Build history of the part. All positions in model axes, mm. Face numbers are marked on the shaded views. A direction names the side the tool comes from. Coordinates: 2 decimals unless noted, no trailing zeros. Loops run counter-clockwise (first coordinate to the right, second up) from the corner with the lowest first, then second, coordinate; pieces in that order, holes last.
Item 1: Cut at B-B (z = 5.25). List the corners of the cut face in (x, y).
Item 2: Cut at A-A (y = 5.5). List the corners of the cut face in (x, z), and give its area (3 significant figures).
Item 3: Flat gauge pin, fed straight in: pin 1 (0.8 mm diameter, centred on x = 8, z = 5.5, fed in from -Y). Where does the tip first touch, or does it go through?
Item 4: Cut at C-C (x = 4.5). List the corners of the cut face in (y, z), and give its area (3 significant figures).
Item 5: Mould opens along X. For the marked faces 1, 2, 3 and 4 say: released by +X, released by -X, zero draft, split by the parting line, or undercut.
Item 6: Drill centre lines: line 1 along X through (y, z) = (-7, 4); line 2 along X through (y, z) = (5, 5); line 3 along Y through (x, z) = (-7, 4). Where is each one in solid material? Low to high.
Item 7: 3-axis set-ups, long thin cutter, end or side, ignore diameter. For the marked faces 5 and 6: which of +Z, -Z, +X, -X, +Y, -Y reach the whole face in a straight line?
Item 8: Cut at D-D (y = -5.25). List the corners of the cut face in (x, z).
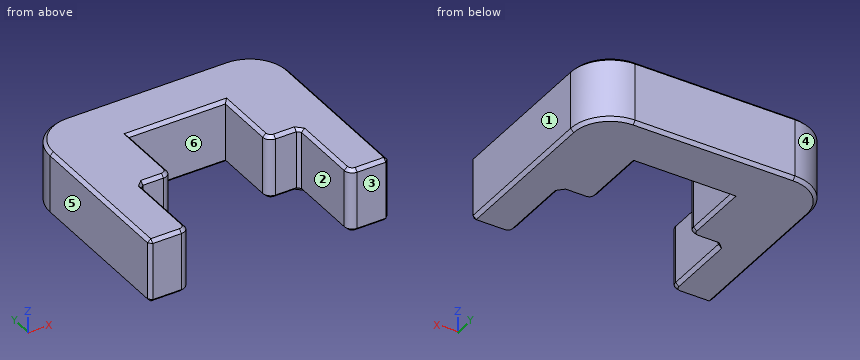
Autodesk Fusion 360 part; units mm, degrees
sketch "Sketch1" plane through (0, 0, 0) normal (0, 0, 1) x (1, 0, 0)
  line L0 (15.05, 12.5) -> (-15.05, 12.5)
  line L1 (-15.05, 12.5) -> (-15.05, -12.5)
  line L2 (-15.05, -12.5) -> (15.05, -12.5)
  line L3 (15.05, -12.5) -> (15.05, 12.5)
  line L4 (15.05, 12.5) -> (-15.05, -12.5) construction
  line L5 (-15.05, 12.5) -> (15.05, -12.5) construction
  line L6 (-10.05, -12.5) -> (-10.05, -2.5)
  line L7 (-10.05, -2.5) -> (-6.05, -2.5)
  line L8 (0, 12.5) -> (0, -12.5) construction
  line L9 (-6.05, -2.5) -> (-6.05, 6)
  line L10 (-6.05, 6) -> (0, 6)
  line L11 (10.05, -12.5) -> (10.05, -2.5)
  line L12 (10.05, -2.5) -> (6.05, -2.5)
  line L13 (6.05, -2.5) -> (6.05, 6)
  line L14 (6.05, 6) -> (0, 6)
  dimension "d2" = 25
  dimension "d3" = 10.05
  dimension "d4" = 10
  dimension "d5" = 6.05
  dimension "d6" = 8.5
  dimension "d12" = 5
extrude "Extrude1" add sketch "Sketch1" along normal blind 8 contours L0 L1 L2 L3 L6 L7 L9 L10 L11 L12 L13 L14
fillet "Fillet1" radius 5 2 edges at (-15.05, 12.5, 4) (15.05, 12.5, 4)
fillet "Fillet2" radius 1 4 edges at (-10.05, -12.5, 4) (-6.05, -2.5, 4) (6.05, -2.5, 4) (10.05, -12.5, 4)
chamfer "Chamfer2" distance 0.4 angle 45 40 edges at (6.05, 2.25, 0) (6.3429, -2.2071, 0) (8.55, -2.5, 0) (0, 6, 0) (-8.55, -2.5, 0) (-6.3429, -2.2071, 0) (-6.05, 2.25, 0) (-13.05, -12.5, 0) (-10.3429, -12.2071, 0) (-10.05, -7, 0) (10.05, -7, 0) (10.3429, -12.2071, 0) (13.05, -12.5, 0) (15.05, -12.5, 4) (13.05, -12.5, 8) (10.3429, -12.2071, 8) (10.05, -7, 8) (-15.05, -12.5, 4) (-10.05, -7, 8) (-10.3429, -12.2071, 8) (-13.05, -12.5, 8) (-6.05, 2.25, 8) (-6.3429, -2.2071, 8) (-8.55, -2.5, 8) (0, 6, 8) (8.55, -2.5, 8) (6.3429, -2.2071, 8) (6.05, 2.25, 8) (15.05, -2.5, 8) (13.5855, 11.0355, 8) (0, 12.5, 8) (-13.5855, 11.0355, 8) (-15.05, -2.5, 8) (15.05, -2.5, 0) (13.5855, 11.0355, 0) (0, 12.5, 0) (-13.5855, 11.0355, 0) (-15.05, -2.5, 0) (-10.05, -2.5, 4) (10.05, -2.5, 4)
Filled sheet:
1. outline: (-15.05, -12.1) - (-14.65, -12.5) - (-11.05, -12.5) arc R1 ccw to (-10.05, -11.5) - (-10.05, -2.9) - (-9.65, -2.5) - (-7.05, -2.5) arc R1 ccw to (-6.05, -1.5) - (-6.05, 6) - (6.05, 6) - (6.05, -1.5) arc R1 ccw to (7.05, -2.5) - (9.65, -2.5) - (10.05, -2.9) - (10.05, -11.5) arc R1 ccw to (11.05, -12.5) - (14.65, -12.5) - (15.05, -12.1) - (15.05, 7.5) arc R5 ccw to (10.05, 12.5) - (-10.05, 12.5) arc R5 ccw to (-15.05, 7.5) - close
2. outline: (-15.05, 0.4) - (-14.65, 0) - (-6.45, 0) - (-6.05, 0.4) - (-6.05, 7.6) - (-6.45, 8) - (-14.65, 8) - (-15.05, 7.6) - close; (6.05, 0.4) - (6.45, 0) - (14.65, 0) - (15.05, 0.4) - (15.05, 7.6) - (14.65, 8) - (6.45, 8) - (6.05, 7.6) - close
2. area: 143 mm2
3. pin 1: stops at y = -2.5
4. outline: (6, 0.4) - (6.4, 0) - (12.1, 0) - (12.5, 0.4) - (12.5, 7.6) - (12.1, 8) - (6.4, 8) - (6, 7.6) - close
4. area: 51.7 mm2
5. face 1: released by +X
5. face 2: undercut
5. face 3: zero draft
5. face 4: released by -X
6. line 1: x = -15.05 to -10.05, 10.05 to 15.05
6. line 2: x = -15.05 to -6.05, 6.05 to 15.05
6. line 3: y = -2.5 to 12.5
7. face 5: +Z, -Z, -X, +Y, -Y
7. face 6: +Z, -Z, -Y
8. outline: (-15.05, 0.4) - (-14.65, 0) - (-10.45, 0) - (-10.05, 0.4) - (-10.05, 7.6) - (-10.45, 8) - (-14.65, 8) - (-15.05, 7.6) - close; (10.05, 0.4) - (10.45, 0) - (14.65, 0) - (15.05, 0.4) - (15.05, 7.6) - (14.65, 8) - (10.45, 8) - (10.05, 7.6) - close
